```python
from build123d import *

# Parameters (mm, degrees)
SKETCH1_R           = 2.6035
BOSS_EXTRUDE1_DEPTH = 304.8


with BuildPart() as part:
    # Sketch1 → Boss-Extrude1 (new body)
    with BuildSketch(Plane(origin=(0, 0, -304.8), x_dir=(-1, 0, 0), z_dir=(0, 0, -1))):
        with BuildLine():
            Line((6.416409763, -10.4902), (4.28752, -10.4902))
            ThreePointArc((4.28752, -10.4902), (3.545750844, -10.797450844), (3.2385, -11.53922))
            Line((3.2385, -11.53922), (3.2385, -11.65098))
            ThreePointArc((3.2385, -11.65098), (3.545750844, -12.392749156), (4.28752, -12.7))
            Line((4.28752, -12.7), (5.3170836, -12.7))
            ThreePointArc((5.3170836, -12.7), (5.8250836, -12.192), (6.3330836, -12.7))
            Line((6.3330836, -12.7), (9.5504, -12.7))
            ThreePointArc((9.5504, -12.7), (10.058323491, -12.192000006), (10.566399977, -12.699846982))
            ThreePointArc((10.566399977, -12.699846982), (12.082522516, -12.082522516), (12.699846982, -10.566399977))
            ThreePointArc((12.699846982, -10.566399977), (12.192000006, -10.058323491), (12.7, -9.5504))
            Line((12.7, -9.5504), (12.7, -6.3330836))
            ThreePointArc((12.7, -6.3330836), (12.192, -5.8250836), (12.7, -5.3170836))
            Line((12.7, -5.3170836), (12.7, 5.3171344))
            ThreePointArc((12.7, 5.3171344), (12.192, 5.8251344), (12.7, 6.3331344))
            Line((12.7, 6.3331344), (12.7, 9.5504))
            ThreePointArc((12.7, 9.5504), (12.192000006, 10.058323491), (12.699846982, 10.566399977))
            ThreePointArc((12.699846982, 10.566399977), (12.082522516, 12.082522516), (10.566399977, 12.699846982))
            ThreePointArc((10.566399977, 12.699846982), (10.058323491, 12.192000006), (9.5504, 12.7))
            Line((9.5504, 12.7), (6.3331344, 12.7))
            ThreePointArc((6.3331344, 12.7), (5.8251344, 12.192), (5.3171344, 12.7))
            Line((5.3171344, 12.7), (4.2874692, 12.7))
            ThreePointArc((4.2874692, 12.7), (3.545700044, 12.392749156), (3.2384492, 11.65098))
            Line((3.2384492, 11.65098), (3.2384492, 11.53922))
            ThreePointArc((3.2384492, 11.53922), (3.545700044, 10.797450844), (4.2874692, 10.4902))
            Line((4.2874692, 10.4902), (6.416384363, 10.4902))
            ThreePointArc((6.416384363, 10.4902), (7.355223148, 9.862578342), (7.134149423, 8.755124678))
            Line((7.134149423, 8.755124678), (3.796632915, 5.423689619))
            ThreePointArc((3.796632915, 5.423689619), (2.767299421, 4.736928798), (1.553617102, 4.4958))
            Line((1.553617102, 4.4958), (-1.657299581, 4.4958))
            ThreePointArc((-1.657299581, 4.4958), (-2.8709819, 4.736928798), (-3.900315394, 5.423689619))
            Line((-3.900315394, 5.423689619), (-7.207191475, 8.724540082))
            ThreePointArc((-7.207191475, 8.724540082), (-7.43216212, 9.851515102), (-6.476774195, 10.4902))
            Line((-6.476774195, 10.4902), (-4.2874692, 10.4902))
            ThreePointArc((-4.2874692, 10.4902), (-3.545700044, 10.797450844), (-3.2384492, 11.53922))
            Line((-3.2384492, 11.53922), (-3.2384492, 11.65098))
            ThreePointArc((-3.2384492, 11.65098), (-3.545700044, 12.392749156), (-4.2874692, 12.7))
            Line((-4.2874692, 12.7), (-5.3170836, 12.7))
            ThreePointArc((-5.3170836, 12.7), (-5.8250836, 12.192), (-6.3330836, 12.7))
            Line((-6.3330836, 12.7), (-9.5504, 12.7))
            ThreePointArc((-9.5504, 12.7), (-10.058323491, 12.192000006), (-10.566399977, 12.699846982))
            ThreePointArc((-10.566399977, 12.699846982), (-12.082522516, 12.082522516), (-12.699846982, 10.566399977))
            ThreePointArc((-12.699846982, 10.566399977), (-12.192000006, 10.058323491), (-12.7, 9.5504))
            Line((-12.7, 9.5504), (-12.7, 6.3331344))
            ThreePointArc((-12.7, 6.3331344), (-12.192, 5.8251344), (-12.7, 5.3171344))
            Line((-12.7, 5.3171344), (-12.7, 4.287470133))
            ThreePointArc((-12.7, 4.287470133), (-12.392749156, 3.545700977), (-11.65098, 3.238450133))
            Line((-11.65098, 3.238450133), (-11.53922, 3.238450133))
            ThreePointArc((-11.53922, 3.238450133), (-10.797450844, 3.545700977), (-10.4902, 4.287470133))
            Line((-10.4902, 4.287470133), (-10.4902, 6.402089023))
            ThreePointArc((-10.4902, 6.402089023), (-9.856394933, 7.351113629), (-8.736962546, 7.129240479))
            Line((-8.736962546, 7.129240479), (-5.440484187, 3.838768792))
            ThreePointArc((-5.440484187, 3.838768792), (-4.75073678, 2.808015636), (-4.5085, 1.591658411))
            Line((-4.5085, 1.591658411), (-4.5085, -1.591658411))
            ThreePointArc((-4.5085, -1.591658411), (-4.75073678, -2.808015636), (-5.440484187, -3.838768792))
            Line((-5.440484187, -3.838768792), (-8.736962546, -7.129240479))
            ThreePointArc((-8.736962546, -7.129240479), (-9.856394933, -7.351113629), (-10.4902, -6.402089023))
            Line((-10.4902, -6.402089023), (-10.4902, -4.287470133))
            ThreePointArc((-10.4902, -4.287470133), (-10.797450844, -3.545700977), (-11.53922, -3.238450133))
            Line((-11.53922, -3.238450133), (-11.65098, -3.238450133))
            ThreePointArc((-11.65098, -3.238450133), (-12.392749156, -3.545700977), (-12.7, -4.287470133))
            Line((-12.7, -4.287470133), (-12.7, -5.3170836))
            ThreePointArc((-12.7, -5.3170836), (-12.192, -5.8250836), (-12.7, -6.3330836))
            Line((-12.7, -6.3330836), (-12.7, -9.5504))
            ThreePointArc((-12.7, -9.5504), (-12.192000006, -10.058323491), (-12.699846982, -10.566399977))
            ThreePointArc((-12.699846982, -10.566399977), (-12.082522516, -12.082522516), (-10.566399977, -12.699846982))
            ThreePointArc((-10.566399977, -12.699846982), (-10.058323491, -12.192000006), (-9.5504, -12.7))
            Line((-9.5504, -12.7), (-6.3331344, -12.7))
            ThreePointArc((-6.3331344, -12.7), (-5.8251344, -12.192), (-5.3171344, -12.7))
            Line((-5.3171344, -12.7), (-4.28752, -12.7))
            ThreePointArc((-4.28752, -12.7), (-3.545750844, -12.392749156), (-3.2385, -11.65098))
            Line((-3.2385, -11.65098), (-3.2385, -11.53922))
            ThreePointArc((-3.2385, -11.53922), (-3.545750844, -10.797450844), (-4.28752, -10.4902))
            Line((-4.28752, -10.4902), (-6.40834956, -10.4902))
            ThreePointArc((-6.40834956, -10.4902), (-7.350269456, -9.860518594), (-7.128470204, -8.749430454))
            Line((-7.128470204, -8.749430454), (-3.796658315, -5.423689619))
            ThreePointArc((-3.796658315, -5.423689619), (-2.767324821, -4.736928798), (-1.553642502, -4.4958))
            Line((-1.553642502, -4.4958), (1.553642502, -4.4958))
            ThreePointArc((1.553642502, -4.4958), (2.767324821, -4.736928798), (3.796658315, -5.423689619))
            Line((3.796658315, -5.423689619), (7.134174823, -8.755124678))
            ThreePointArc((7.134174823, -8.755124678), (7.355248548, -9.862578342), (6.416409763, -10.4902))
        make_face()
        Circle(SKETCH1_R, mode=Mode.SUBTRACT)
        with BuildLine():
            Line((10.4902, 6.446436794), (10.4902, -6.425372487))
            ThreePointArc((10.4902, -6.425372487), (9.862352148, -7.36547709), (8.753441447, -7.145689354))
            Line((8.753441447, -7.145689354), (5.440484187, -3.838768792))
            ThreePointArc((5.440484187, -3.838768792), (4.75073678, -2.808015636), (4.5085, -1.591658411))
            Line((4.5085, -1.591658411), (4.5085, 1.591658411))
            ThreePointArc((4.5085, 1.591658411), (4.75073678, 2.808015636), (5.440484187, 3.838768792))
            Line((5.440484187, 3.838768792), (8.768349738, 7.160570479))
            ThreePointArc((8.768349738, 7.160570479), (9.867741577, 7.378471563), (10.4902, 6.446436794))
        make_face(mode=Mode.SUBTRACT)
    extrude(amount=-BOSS_EXTRUDE1_DEPTH)


solid = part.part
```
Geometry: final body of the model. Coordinates: model frame, mm. Give positions to 0.01 mm unless a question says otherwise; leave off trailing zeros. Answer as CSV lines item,"result". Start each with the question number.
1) Mould query, pull axis Y, two halves, no side actions, for faces 1 (the flat face through (-12.7, 0, -155)), 2 (the flat face through (-10.49, 0, -155)). Classes: +Y half, -Y half, draft (parallel to the pull), parting line (faces both ways), or undercut.
2) First-contact query: P1, Ø1, axis at x = 0.5, z = -166, coming from the +Y side; P2, Ø1, axis at y = -0.5, z = -133, coming from the +X side; P3, Ø1.6, axis at x = -0.5, z = -180.5, coming from the -Y side. Flat tips, straight axial feed; report the tip coordinate or a pass-through.
3) Line query: line 1 (X direction, y = 0.5, z = -211); line 2 (X direction, y = 6.25, z = -37); line 3 (Y direction, x = 0, z = -210). Output: solid intervals per line, ascending. Write a range as from..to.
4) Cut plane A-A (z = -98). State how many separate pieces and enclosed holes the cut face has, then the cut area to 3 significant figures.
Findings below:
1,face 1,"draft"
1,face 2,"undercut"
2,P1,"stops at y = 4.5"
2,P2,"stops at x = 4.51"
2,P3,"stops at y = -4.5"
3,line 1,"x = -12.7..-10.49, -4.51..-2.56, 2.56..4.51"
3,line 2,"x = -12.42..-10.49, -7.86..-4.62, 4.73..7.86, 10.49..12.42"
3,line 3,"y = -4.5..-2.6, 2.6..4.5"
4,separate pieces,"1"
4,enclosed holes,"2"
4,area,"297 mm²"
